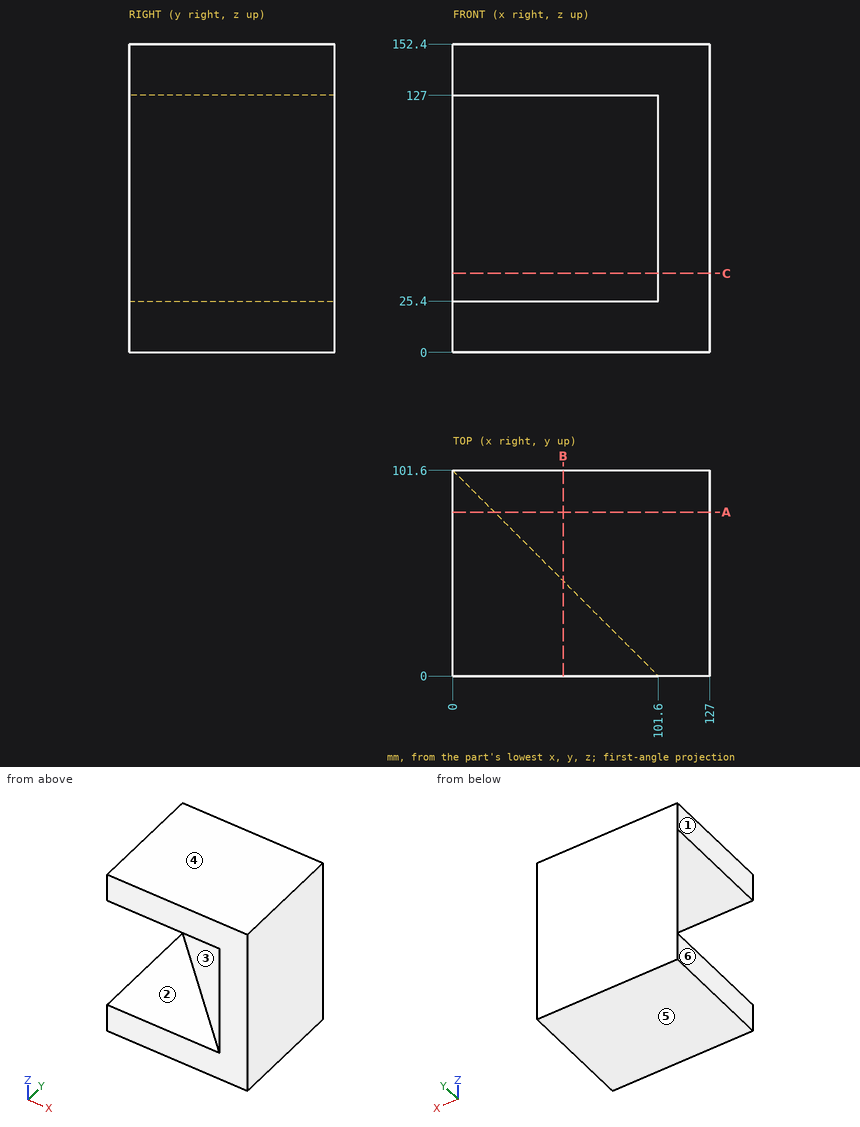
Input: dimensioned drawing with shaded views. Units: mm. Origin: part minimum x, y, z. A direction names the side the tool comes from. Coordinates: 2 decimals unless noted, no trailing zeros. Loops run counter-clockwise (first coordinate to the right, second up) from the corner with the lowest first, then second, coordinate; pieces in that order, holes last.
Q1. Section B-B, the plane x = 54.5. Return the cut outline in (y, z).
Results are:
outline: (0, 0) - (101.6, 0) - (101.6, 152.4) - (0, 152.4) - (0, 127) - (47.1, 127) - (47.1, 25.4) - (0, 25.4) - close
Q2. Set-up query: the marked faces 1 and 2. Return all of +Z, -Z, +X, -X, +Y, -Y with unobstructed straight access to the full face (end or side cutting, diameter ignored); none if empty.
Results are:
face 1: +Z, -Z, -X, +Y, -Y
face 2: -X, -Y
Q3. Mould query, pull axis Z, two halves, no side actions, for the marked faces 3, 4, 5 and 6. Classes: +Z half, -Z half, draft (parallel to the pull), parting line (faces both ways), or undercut.
Results are:
face 3: undercut
face 4: +Z half
face 5: -Z half
face 6: draft
Q4. Section A-A, the plane y = 81. Return the cut outline in (x, z), and give its area (3 significant figures).
Results are:
outline: (0, 0) - (127, 0) - (127, 152.4) - (0, 152.4) - (0, 127) - (20.6, 127) - (20.6, 25.4) - (0, 25.4) - close
area: 17,300 mm2
Q5. Section C-C, the plane z = 39. Return the cut outline in (x, y).
Results are:
outline: (0, 101.6) - (101.6, 0) - (127, 0) - (127, 101.6) - close
Q6. Contact query for flat-ended pins moving along their axis: pin 1 (2 mm diameter, centred on x = 89.5, z = 48, fed in from -Y); pin 2 (3 mm diameter, centred on x = 53, z = 41.5, fed in from -Y); pin 3 (1.5 mm diameter, centred on x = 87.5, z = 33.5, fed in from -Y). Output: stop coordinate, or through.
Results are:
pin 1: stops at y = 11.1
pin 2: stops at y = 47.1
pin 3: stops at y = 13.35
Q7. Line query: line 1 along Z through (x, y) = (59, 39.5); line 2 along Y through (x, z) = (30, 34); line 3 along X through (y, z) = (78.5, 123). Output: solid intervals per line, ascending.
Results are:
line 1: z = 0 to 25.4, 127 to 152.4
line 2: y = 71.6 to 101.6
line 3: x = 23.1 to 127
